Model file for the job. Use its own axes, mm. A direction names the side the tool comes from. Round coordinates to 2 decimals unless told otherwise and drop trailing zeros. Order: outer loops, then holes, each group sorted by start corner. A loop starts at its lowest first (then second) coordinate and runs counter-clockwise, first axis right, second up. Notation, with made-up numbers: (39, 57.25) -> (72, 57.25) arc R32 ccw to (72, 94.25) -> close; hole circle Ø10 at (49, -12.75). An arc over 180 degrees is marked (long way). Use CSV: the item, a comma, the result in double quotes.
```python
from build123d import *

# Parameters (mm, degrees)
EXTRUDE_1_DEPTH    = 17
HOLE_WIZARD_M3_1_D = 2.5
SKETCH_4_R         = 1.5
EXTRUDE_2_DEPTH    = 6


with BuildPart() as part:
    # 草图1 → 凸台-拉伸1 (new body)
    with BuildSketch(Plane.XY):
        Polygon((0, 0), (2.5, 0), (3.75, -2.165063509), (2.5, -4.330127019), (0, -4.330127019), (-1.25, -2.165063509), align=None)
    extrude(amount=EXTRUDE_1_DEPTH)

    # M3 螺纹孔1 (through all)
    with Locations(Plane.XY.offset(17)):
        with Locations((1.25, -2.165063509)):
            Hole(HOLE_WIZARD_M3_1_D / 2)

    # 草图4 → 凸台-拉伸2 (add)
    with BuildSketch(Plane.XY.offset(17)):
        with Locations(Location((1.25, -2.165063509, 0), (0, 0, 180))):
            Circle(SKETCH_4_R)
    extrude(amount=EXTRUDE_2_DEPTH)


solid = part.part
```
Q1. Probe line 1 along Y through (x, z) = (1.25, 10); line 2 along X through (y, z) = (-3.2, 16.25); line 3 along Z through (x, y) = (2.6, -3.1). List the from-to ranges inside material, lowest first.
From the geometry:
line 1,"y = -4.33 to -3.42, -0.92 to 0"
line 2,"x = -0.65 to 0.55, 1.95 to 3.15"
line 3,"z = 0 to 17"
Q2. Cut at A-A (x = 1.25). Give the cut face in (y, z).
From the geometry:
outline,"(-4.33, 0) -> (-3.42, 0) -> (-3.42, 17) -> (-0.92, 17) -> (-0.92, 0) -> (0, 0) -> (0, 17) -> (-0.67, 17) -> (-0.67, 23) -> (-3.67, 23) -> (-3.67, 17) -> (-4.33, 17) -> close"
Q3. Pin check, flat tip, straight feed: pin 1 (0.8 mm diameter, centred on x = 2, y = -2, fed in from -Z). Stop position of the tip, or through.
From the geometry:
pin 1,"stops at z = 17"
Q4. Mould opens along Y. For faces 3 (the cylindrical face through (0.058, -1.79, 8.381)), 4 (the cylindrical face through (2.356, -3.179, 19.958)), 5 (the flat face through (1, -2, 17)), 6 (the flat face through (3.12, -1.07, 8.38)) say: +Y half, -Y half, draft (parallel to the pull), parting line (faces both ways), or undercut.
From the geometry:
face 3,"undercut"
face 4,"parting line"
face 5,"undercut"
face 6,"+Y half"
Q5. Cut at B-B (z = 3.75). Give the cut face in (x, y).
From the geometry:
outline,"(-1.25, -2.17) -> (0, -4.33) -> (2.5, -4.33) -> (3.75, -2.17) -> (2.5, 0) -> (0, 0) -> close; hole circle Ø2.5 at (1.25, -2.17)"
Q6. Which spindle directions (+Z, -Z, +X, -X, +Y, -Y) get a long thin tool onto all of the face, cutting with end or side? Do faces 1 (the flat face through (-0.634, -1.098, 8.381)), 2 (the flat face through (-0.4, -2.1, 17)). Say none if no direction does.
From the geometry:
face 1,"+Z, -Z, -X, +Y"
face 2,"+Z"
Q7. Cut at C-C (y = -2.7). Give the cut face in (x, z).
From the geometry:
outline,"(-0.94, 0) -> (0.12, 0) -> (0.12, 17) -> (2.38, 17) -> (2.38, 0) -> (3.44, 0) -> (3.44, 17) -> (2.65, 17) -> (2.65, 23) -> (-0.15, 23) -> (-0.15, 17) -> (-0.94, 17) -> close"
